Study the drawing (mm; zero at the part's minimum x, y, z) and answer. Round coordinates to 2 decimals unless told otherwise and drop trailing zeros. Loops run counter-clockwise (first coordinate to the right, second up) from the corner with the lowest first, then second, coordinate; pieces in that order, holes last. Notation, with made-up numbers: (70.5, 0) -> (91.5, 0) arc R27 ccw to (91.5, 37) -> close; hole circle Ø3 at (26, -1.5). An arc over 180 degrees is marked (long way). Write each question's results on one line, items separated by ' | '. Start each with the question number.
(1) The part is cut by section A-A (z = 10.05). Determine the outline of the cut face in (x, y).
(2) Straight lines are drawn through the part: probe 1 along Z at (x, y) = (4, 10.05); probe 2 along Z at (x, y) = (16.5, 10.05). For each, find the intervals that lie inside material, in ascending order.
(3) Determine the mould class of the marked faces 1, 2, 3 and 4 for opening direction Y: released by +Y, released by -Y, zero draft, split by the parting line, or undercut.
(4) The part is cut by section D-D (y = 13.25). Determine the outline of the cut face in (x, z).
(5) Flat-ended cylindrical pins translate along their axes: pin 1 (1.5 mm diameter, centred on x = 17.5, z = 12, fed in from -Y); pin 2 (6 mm diameter, centred on x = 21.5, z = 6.5, fed in from -Y); pin 3 (1 mm diameter, centred on x = 17, y = 17, fed in from -Z). Find the tip coordinate at first contact, or state that the pin passes through.
(6) The part is cut by section C-C (x = 14). Determine the outline of the cut face in (y, z).
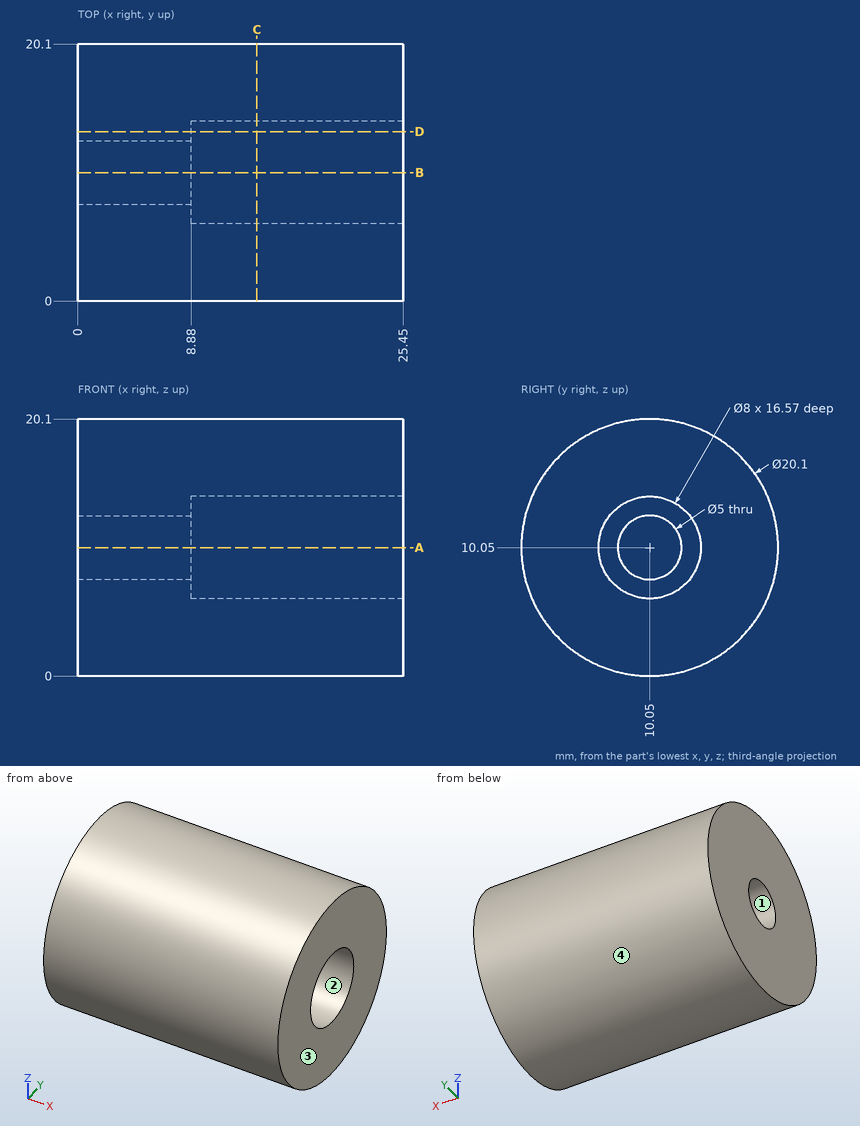
Checked values:
1) outline: (0, 0) -> (25.45, 0) -> (25.45, 6.05) -> (8.88, 6.05) -> (8.88, 7.55) -> (0, 7.55) -> close; (0, 12.55) -> (8.88, 12.55) -> (8.88, 14.05) -> (25.45, 14.05) -> (25.45, 20.1) -> (0, 20.1) -> close
2) probe 1: z = 0 to 7.55, 12.55 to 20.1 | probe 2: z = 0 to 6.05, 14.05 to 20.1
3) face 1: undercut | face 2: undercut | face 3: zero draft | face 4: split by the parting line
4) outline: (0, 0.52) -> (25.45, 0.52) -> (25.45, 7.65) -> (8.88, 7.65) -> (8.88, 12.45) -> (25.45, 12.45) -> (25.45, 19.58) -> (0, 19.58) -> close
5) pin 1: stops at y = 0.07 | pin 2: stops at y = 0.02 | pin 3: stops at z = 2.34
6) outline: circle Ø20.1 at (10.05, 10.05); hole circle Ø8 at (10.05, 10.05)
